```python
from build123d import *

# Parameters (mm, degrees)
SKETCH1_W                      = 231.775
SKETCH1_H                      = 81.4959
BOSS_EXTRUDE1_DEPTH            = 2.38125
F_4_CLEARANCE_HOLE1_D          = 3.2639
F_4_CLEARANCE_HOLE2_AT_2_COUNT = 2
F_4_CLEARANCE_HOLE2_AT_2_PITCH = 12.7
F_1_2_0_5_DIAMETER_HOLE1_D     = 12.7


with BuildPart() as part:
    # Sketch1 → Boss-Extrude1 (new body)
    with BuildSketch(Plane.XY):
        Rectangle(SKETCH1_W, SKETCH1_H)
    extrude(amount=BOSS_EXTRUDE1_DEPTH)

    # #4 Clearance Hole1 (through all)
    with Locations(Plane.XY.offset(2.38125)):
        with Locations((-11.29792, 28.575), (26.80208, 28.575)):
            f_4_clearance_hole1 = Hole(F_4_CLEARANCE_HOLE1_D / 2)

    # Mirror1: #4 Clearance Hole1 across plane
    add(f_4_clearance_hole1.mirror(Plane.ZX), mode=Mode.SUBTRACT)

    # Sketch6 → #4 Clearance Hole2 (revolve, cut)
    with BuildSketch(Plane(origin=(-112.7125, 30.82036, 2.38125), x_dir=(0, -1, 0), z_dir=(1, 0, 0))):
        Polygon((0, 0), (0, 10.505574487), (1.63195, 9.525), (1.63195, 0), align=None)
    f_4_clearance_hole2 = revolve(axis=Axis((-112.7125, 30.82036, 8.73125), (0, 0, -1)), mode=Mode.SUBTRACT)

    # #4 Clearance Hole2 at 2: #4 Clearance Hole2 ×2
    with Locations(*[(i * F_4_CLEARANCE_HOLE2_AT_2_PITCH, 0, 0) for i in range(1, F_4_CLEARANCE_HOLE2_AT_2_COUNT)]):
        add(f_4_clearance_hole2, mode=Mode.SUBTRACT)

    # Mirror2: #4 Clearance Hole2 across plane
    add(f_4_clearance_hole2.mirror(Plane(origin=(0, 0, 0), x_dir=(0, 0, 1), z_dir=(1, 0, 0))), mode=Mode.SUBTRACT)

    # Mirror2 copy 1 sketch → Mirror2 copy 1 (revolve, cut)
    with BuildSketch(Plane(origin=(100.0125, 30.82036, 2.38125), x_dir=(0, -1, 0), z_dir=(-1, 0, 0))):
        Polygon((0, 0), (0, -10.505574487), (1.63195, -9.525), (1.63195, 0), align=None)
    revolve(axis=Axis((100.0125, 30.82036, 8.73125), (0, 0, 1)), mode=Mode.SUBTRACT)

    # Mirror3: #4 Clearance Hole2 across plane
    add(f_4_clearance_hole2.mirror(Plane.ZX), mode=Mode.SUBTRACT)

    # Mirror3 copy 1 sketch → Mirror3 copy 1 (revolve, cut)
    with BuildSketch(Plane(origin=(-100.0125, -30.82036, 2.38125), x_dir=(0, 1, 0), z_dir=(1, 0, 0))):
        Polygon((0, 0), (0, -10.505574487), (1.63195, -9.525), (1.63195, 0), align=None)
    revolve(axis=Axis((-100.0125, -30.82036, 8.73125), (0, 0, 1)), mode=Mode.SUBTRACT)

    # Mirror3 copy 2 sketch → Mirror3 copy 2 (revolve, cut)
    with BuildSketch(Plane(origin=(112.7125, -30.82036, 2.38125), x_dir=(0, 1, 0), z_dir=(-1, 0, 0))):
        Polygon((0, 0), (0, 10.505574487), (1.63195, 9.525), (1.63195, 0), align=None)
    revolve(axis=Axis((112.7125, -30.82036, 8.73125), (0, 0, -1)), mode=Mode.SUBTRACT)

    # Mirror3 copy 3 sketch → Mirror3 copy 3 (revolve, cut)
    with BuildSketch(Plane(origin=(100.0125, -30.82036, 2.38125), x_dir=(0, 1, 0), z_dir=(-1, 0, 0))):
        Polygon((0, 0), (0, 10.505574487), (1.63195, 9.525), (1.63195, 0), align=None)
    revolve(axis=Axis((100.0125, -30.82036, 8.73125), (0, 0, -1)), mode=Mode.SUBTRACT)

    # 1/2 (0.5) Diameter Hole1 (through all)
    with Locations(Plane.XY.offset(2.38125)):
        with Locations((0, 0)):
            Hole(F_1_2_0_5_DIAMETER_HOLE1_D / 2)


solid = part.part
```
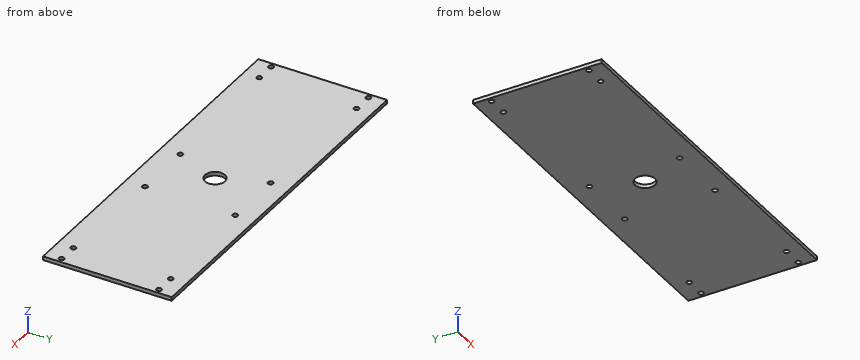
Part model, mm, in its own coordinate system. Coordinates: 2 decimals unless noted, no trailing zeros. Write each loop counter-clockwise with the first axis right and the second up, starting at its lowest first coordinate (ties: lowest second). Pieces come first, ordered by that corner, then holes.
Item 1: Probe line 1 (X direction, y = -27.5, z = 0.7); line 2 (Y direction, x = -12, z = 1.45); line 3 (X direction, y = 1, z = 1.25). List the from-to ranges inside material, lowest first.
Item 2: Slice it at B-B (y = 0). Write the cut outline in (x, z), and give its area (3 significant figures).
Item 3: Slice it at A-A (x = 0). Write the cut outline in (y, z).
Results found:
1. line 1: x = -115.89 to -12.53, -10.07 to 25.57, 28.03 to 115.89
1. line 2: y = -40.75 to -30.05, -27.1 to 27.1, 30.05 to 40.75
1. line 3: x = -115.89 to -6.27, 6.27 to 115.89
2. outline: (-115.89, 0) - (-6.35, 0) - (-6.35, 2.38) - (-115.89, 2.38) - close; (6.35, 0) - (115.89, 0) - (115.89, 2.38) - (6.35, 2.38) - close
2. area: 522 mm2
3. outline: (-40.75, 0) - (-6.35, 0) - (-6.35, 2.38) - (-40.75, 2.38) - close; (6.35, 0) - (40.75, 0) - (40.75, 2.38) - (6.35, 2.38) - close
